```python
from build123d import *

# Parameters (mm, degrees)
F1_START = 347.5
F0_R     = 36
F1_DEPTH = 70
F3_START = 282.5
F2_R     = 25
F3_DEPTH = 195
F4_SIZE2 = 2
F4_SIZE  = 2


with BuildPart() as f1:
    # F0 (on Right) → F1 (new body)
    with BuildSketch(Plane.YZ.offset(F1_START)):
        Circle(F0_R)
    extrude(amount=F1_DEPTH)

    # F2 (on Right) → F3 (join)
    with BuildSketch(Plane.YZ.offset(F3_START)):
        Circle(F2_R)
    extrude(amount=F3_DEPTH)

    # F4
    f4_edges = [f1.edges().sort_by_distance(p)[0] for p in [
        (477.5, -25, 0),
        (282.5, -25, 0),
    ]]
    chamfer(f4_edges, length=F4_SIZE, length2=F4_SIZE2)


solid = f1.part
```
Part model, mm, in its own coordinate system. A direction names the side the tool comes from. Coordinates: 2 decimals unless noted, no trailing zeros. Order: outer loops, then holes, each group sorted by start corner. A loop starts at its lowest first (then second) coordinate and runs counter-clockwise, first axis right, second up. Notation, with made-up numbers: (27, 85) - (84, 85) arc R21 ccw to (84, 118) - close; hole circle Ø3 at (53, 84). An arc over 180 degrees is marked (long way). Return JSON: item names as keys, results as strings. Group by question number.
Item 1: Cut at D-D (y = -28). List the corners of the cut face in (x, z), plus the area to 3 significant figures.
Item 2: Drill centre lines: probe 1 along Z at (x, y) = (412, -1); probe 2 along Y at (x, z) = (291.5, -0.5) (3 decimals); probe 3 along X at (y, z) = (31.5, 13). Where is each one in solid material? Low to high. Write a range as from..to.
Item 3: Pin check, flat tips, straight feed: pin 1 (2 mm diameter, centred on y = 26.5, z = -18.5, fed in from +X); pin 2 (8 mm diameter, centred on x = 345, z = -23, fed in from +Y); pin 3 (1.5 mm diameter, centred on y = -2, z = -27, fed in from -X); pin 4 (12 mm diameter, centred on y = 0.5, z = 24, fed in from +X). Stop position of each tip, or through.
Item 4: Cut at C-C (x = 300). List the corners of the cut face in (y, z), plus the area to 3 significant figures.
Item 5: Cut at A-A (z = 0). List the corners of the cut face in (x, y), plus the area to 3 significant figures.
Item 6: Which spindle directions (+Z, -Z, +X, -X, +Y, -Y) get a long thin tool onto all of the face, cutting with end or side? Do faces 1 (the face through (417.5, -25, -7)), 2 (the face through (347.5, -25, -7)), 3 (the face through (477.5, 0, 0)). Say none if no direction does.
Check values:
{
 "1": {"outline": "(347.5, -22.63) - (417.5, -22.63) - (417.5, 22.63) - (347.5, 22.63) - close", "area": "3,170 mm2"},
 "2": {"probe 1": "z = -35.99..35.99", "probe 2": "y = -24.995..24.995", "probe 3": "x = 347.5..417.5"},
 "3": {"pin 1": "stops at x = 417.5", "pin 2": "stops at y = 30.01", "pin 3": "stops at x = 347.5", "pin 4": "stops at x = 477.5"},
 "4": {"outline": "circle Ø50 at (0, 0)", "area": "1,960 mm2"},
 "5": {"outline": "(282.5, -23) - (284.5, -25) - (347.5, -25) - (347.5, -36) - (417.5, -36) - (417.5, -25) - (475.5, -25) - (477.5, -23) - (477.5, 23) - (475.5, 25) - (417.5, 25) - (417.5, 36) - (347.5, 36) - (347.5, 25) - (284.5, 25) - (282.5, 23) - close", "area": "11,300 mm2"},
 "6": {"face 1": "+X", "face 2": "-X", "face 3": "+Z, -Z, +X, +Y, -Y"}
}
